from build123d import *

# Parameters (mm, degrees)
BOSS_EXTRUDE1_DEPTH      = 9.525
BOSS_EXTRUDE1_DEPTH_BACK = 9.525
CUT_EXTRUDE1_DEPTH       = 373.680910299
CUT_EXTRUDE2_DEPTH       = 373.680910299
SKETCH5_W                = 97.518379051
SKETCH5_H                = 136.419580789
CUT_EXTRUDE3_DEPTH       = 739.741184154
SKETCH6_W                = 75.100700845
SKETCH6_H                = 154.277977479
CUT_EXTRUDE4_DEPTH       = 748.678846608
SKETCH7_R                = 4.7625
CUT_EXTRUDE5_DEPTH       = 254
CUT_EXTRUDE6_DEPTH       = 752.699804454
CUT_EXTRUDE6_DEPTH_BACK  = 752.699804454
SKETCH8_W                = 222.997610285
SKETCH8_H                = 196.30354947
SKETCH9_R                = 1.5875
CUT_EXTRUDE7_DEPTH       = 12.7
CUT_EXTRUDE8_START       = -12.7
SKETCH10_R               = 1.5875
CUT_EXTRUDE8_DEPTH       = 12.7


with BuildPart() as part:
    # Sketch1 → Boss-Extrude1 (new, two sides: drawn at the far end of the back side and taken through both)
    with BuildSketch(Plane.XY.offset(-BOSS_EXTRUDE1_DEPTH_BACK)):
        Polygon((101.792411443, 735.656458749), (49.404911443, 673.557276224), (49.404911443, 396.497366015), (154.179911443, 396.497366015), (154.179911443, 556.636391043), (128.683999881, 589.063224066), (151.148766449, 589.063224066), (128.683999881, 617.634912224), (151.148766449, 617.634912224), (129.452026088, 645.229790529), (151.148766449, 645.229790529), (128.876006433, 673.557276224), (154.179911443, 673.557276224), align=None)
    extrude(amount=BOSS_EXTRUDE1_DEPTH + BOSS_EXTRUDE1_DEPTH_BACK)

    # Sketch2 → Cut-Extrude1 (cut, through all)
    with BuildSketch(Plane(origin=(0, 396.497366015, 0), x_dir=(-1, 0, 0), z_dir=(0, -1, 0))):
        Polygon((-49.404911443, 0), (-101.792411443, -9.525), (-154.179911443, 0), (-159.65732669, 0), (-159.65732669, -13.649148588), (-44.158493861, -13.649148588), (-44.158493861, 0), align=None)
    extrude(amount=-CUT_EXTRUDE1_DEPTH, mode=Mode.SUBTRACT)

    # Sketch3 → Cut-Extrude2 (cut, through all)
    with BuildSketch(Plane.XZ.offset(-396.497366015)):
        Polygon((49.404911443, 0), (101.792411443, -9.525), (154.179911443, 0), (159.580570647, 0), (159.580570647, -14.500746269), (43.682013433, -14.500746269), (43.682013433, 0), align=None)
    extrude(amount=-CUT_EXTRUDE2_DEPTH, mode=Mode.SUBTRACT)

    # Sketch5 → Cut-Extrude3 (cut, through all)
    with BuildSketch(Plane(origin=(26.430459561, 22.297003663, 133.782021979), x_dir=(0.9815360247212257, -0.031445805879602766, -0.1886748352776165), z_dir=(0.1912773697394791, 0.16136352846789567, 0.9681811708073739))):
        with Locations((89.248369642, 700.742830845)):
            Rectangle(SKETCH5_W, SKETCH5_H)
    cut_extrude3 = extrude(amount=CUT_EXTRUDE3_DEPTH, mode=Mode.SUBTRACT)

    # Sketch6 → Cut-Extrude4 (cut, through all)
    with BuildSketch(Plane(origin=(-18.981895096, 16.01331916, 96.079914958), x_dir=(0.9815360247212258, 0.03144580587960229, 0.18867483527761636), z_dir=(-0.19127736973947887, 0.1613635284678934, 0.9681811708073744))):
        with Locations((98.873573013, 697.792784398)):
            Rectangle(SKETCH6_W, SKETCH6_H)
    cut_extrude4 = extrude(amount=CUT_EXTRUDE4_DEPTH, mode=Mode.SUBTRACT)

    # Mirror1: Cut-Extrude3, Cut-Extrude4 across plane
    add(cut_extrude3.mirror(Plane.XY), mode=Mode.SUBTRACT)
    add(cut_extrude4.mirror(Plane.XY), mode=Mode.SUBTRACT)

    # Sketch7 → Cut-Extrude5 (cut)
    with BuildSketch(Plane.XZ.offset(-396.497366015)):
        with Locations(Location((101.792411443, 0, 0), (0, 0, 270))):
            Circle(SKETCH7_R)
    extrude(amount=-CUT_EXTRUDE5_DEPTH, mode=Mode.SUBTRACT)

    # Sketch8 → Cut-Extrude6 (cut, two sides: drawn at the far end of the back side and taken through both)
    with BuildSketch(Plane.XY.offset(-CUT_EXTRUDE6_DEPTH_BACK)):
        with Locations((89.854155539, 664.228687117)):
            Rectangle(SKETCH8_W, SKETCH8_H)
    extrude(amount=CUT_EXTRUDE6_DEPTH + CUT_EXTRUDE6_DEPTH_BACK, mode=Mode.SUBTRACT)

    # Sketch9 → Cut-Extrude7 (cut)
    with BuildSketch(Plane(origin=(0, 566.076912382, 0), x_dir=(1, 0, 0), z_dir=(0, 1, 0))):
        with Locations(Location((89.092411443, 0, 0), (0, 0, 270))):
            Circle(SKETCH9_R)
        with Locations(Location((114.492411443, 0, 0), (0, 0, 270))):
            Circle(SKETCH9_R)
    extrude(amount=-CUT_EXTRUDE7_DEPTH, mode=Mode.SUBTRACT)

    # Sketch10 → Cut-Extrude8 (cut)
    with BuildSketch(Plane.XZ.offset(-396.497366015).offset(CUT_EXTRUDE8_START)):
        with Locations(Location((89.092411443, 0, 0), (0, 0, 90))):
            Circle(SKETCH10_R)
        with Locations(Location((114.492411443, 0, 0), (0, 0, 90))):
            Circle(SKETCH10_R)
    extrude(amount=CUT_EXTRUDE8_DEPTH, mode=Mode.SUBTRACT)


solid = part.part
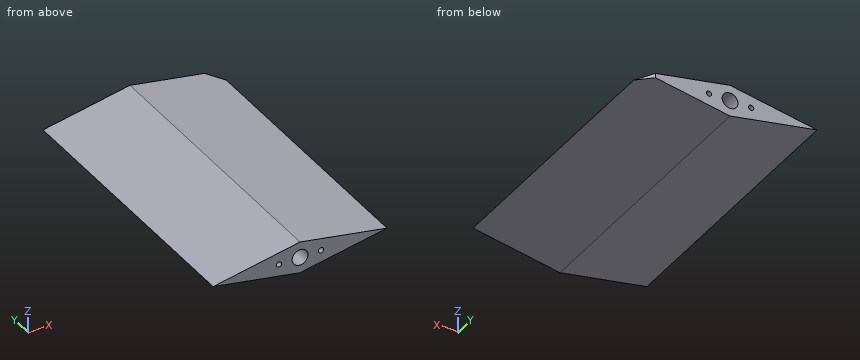
Here's how the part is built. I have some questions about the finished solid (model axes, mm). Round coordinates to 2 decimals unless told otherwise and drop trailing zeros. Loops run counter-clockwise (first coordinate to the right, second up) from the corner with the lowest first, then second, coordinate; pieces in that order, holes last. Notation, with made-up numbers: M 75.25,68 L 83.25,68 A6 cw 83.25,75 Z; hole C 11.5,-35.5 d9. An arc over 180 degrees is marked long. Write each question's results on one line, items separated by ' | '. Start each with the question number.
(1) I want a section at A-A (y = 442.5). Please give me the cut outline in (x, z) (1 decimal), then the cut area to 3 significant figures.
(2) If I drill on probe 1 along Z at (x, y) = (98, 548); probe 2 along Z at (x, y) = (131, 505); probe 3 along Z at (x, y) = (99.5, 414), over which ranges is the centre line in solid material (lowest first)? Write a range as from..to.
(3) I want a section at B-B (x = 136.5). Please give me the cut outline in (y, z).
(4) Will these pins go through, and if not, where does the flat tip stop? P1, Ø1, axis at x = 115, z = -0.5, coming from the +Y side; P2, Ø1.5, axis at x = 136, y = 546.5, coming from the -Z side; P3, Ø1, axis at x = 71, y = 462.5, coming from the +Z side.
(5) I want a section at C-C (z = 6.5). Please give me the cut outline in (x, y), then the cut area to 3 significant figures.
Solved:
1) outline: M 49.4,0 L 101.8,-9.5 L 154.2,0 L 101.8,9.5 Z; hole C 101.8,0 d9.5 | area: 927 mm²
2) probe 1: z = -8.84..-2.88, 2.88..8.84 | probe 2: z = -4.21..4.21 | probe 3: z = -9.11..-4.17, 4.17..9.11
3) outline: M 396.5,-3.21 L 566.08,-3.21 L 566.08,3.21 L 396.5,3.21 Z
4) P1: stops at y = 553.38 | P2: stops at z = -3.44 | P3: stops at z = 4.02
5) outline: M 85.15,396.5 L 118.43,396.5 L 118.43,566.08 L 85.15,566.08 Z | area: 5,640 mm²
